Design review of the part shown in the three views and the two pictorial views. Dimensions are in mm from the part's minimum x, y and z. A direction names the side the tool comes from. Give positions to 0.01 mm unless a question says otherwise; leave off trailing zeros. Loops run counter-clockwise (first coordinate to the right, second up) from the corner with the lowest first, then second, coordinate; pieces in that order, holes last. Notation, with made-up numbers: (-21, 14) -> (-14, 14) arc R12 cw to (-14, 32) -> close; hole circle Ø5 at (24.5, -15). An arc over 180 degrees is marked (long way). Use CSV: the item, a comma, the result in double quotes. Start each with the question number.
Item 1: We need section B-B (y = 36). State the section outline as (x, z) points, plus the area to 3 significant figures.
Item 2: Wall thickness on line 1 along X through (y, z) = (45.72, 11.25); line 2 along X through (y, z) = (18.5, 1.75): over which ranges is each line inside the solid? List them lowest first. Write a range as from..to.
Item 3: We need section D-D (x = 45.72). State the section outline as (y, z) points, plus the area to 3 significant figures.
Item 4: We need section C-C (z = 14). Count the separate pieces of the cut face and the enclosed holes in it, plus the area to 3 significant figures.
Item 5: The part is to be moulded in two halves that separate along X. For the marked faces 1, 2, 3 and 4, say which applies: +X half, -X half, draft (parallel to the pull), parting line (faces both ways), or undercut.
Item 6: For the marked faces 5 and 6, list the 3-axis set-ups (+Z, -Z, +X, -X, +Y, -Y) from which the entire face can be reached by the end or side of a thin tool; tool diameter is ignored.
Item 7: We need section A-A (x = 22.4). State the section outline as (y, z) points.
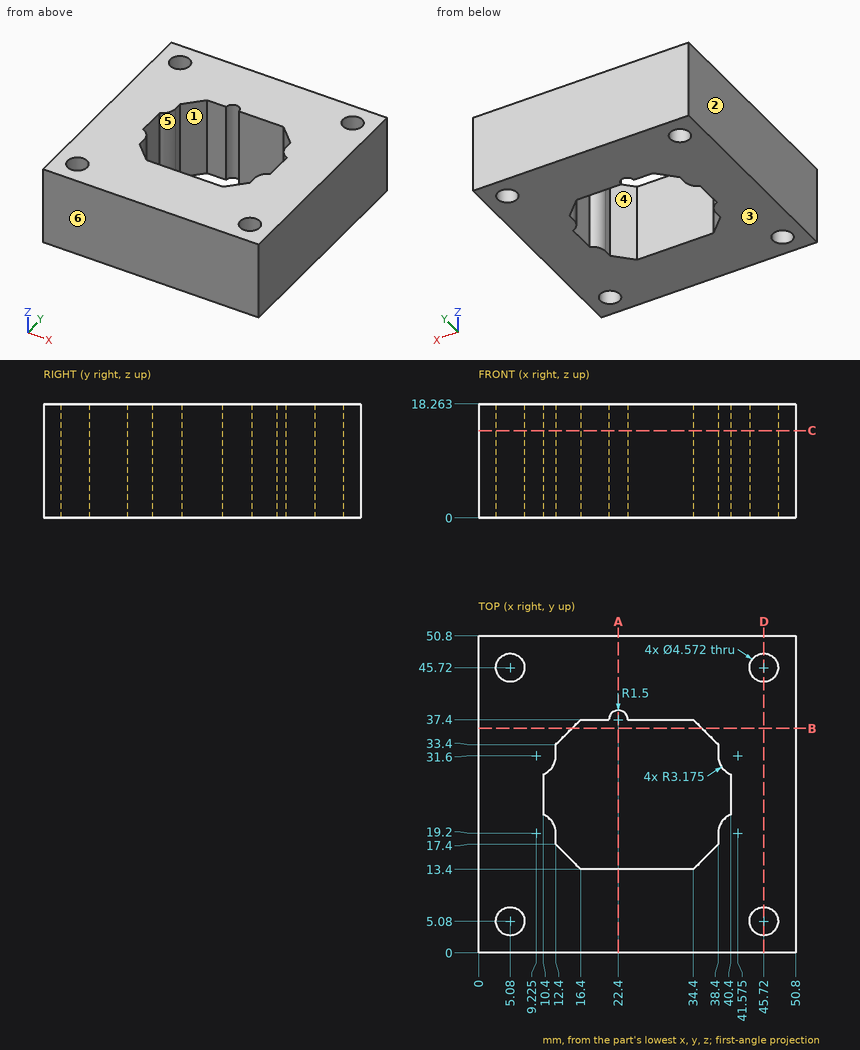
Results found:
1,outline,"(0, 0) -> (15, 0) -> (15, 18.26) -> (0, 18.26) -> close; (35.8, 0) -> (50.8, 0) -> (50.8, 18.26) -> (35.8, 18.26) -> close"
1,area,"548 mm²"
2,line 1,"0..2.79, 7.37..43.43, 48.01..50.8"
2,line 2,"0..12.4, 38.4..50.8"
3,outline,"(0, 0) -> (2.79, 0) -> (2.79, 18.26) -> (0, 18.26) -> close; (7.37, 0) -> (43.43, 0) -> (43.43, 18.26) -> (7.37, 18.26) -> close; (48.01, 0) -> (50.8, 0) -> (50.8, 18.26) -> (48.01, 18.26) -> close"
3,area,"761 mm²"
4,separate pieces,"1"
4,enclosed holes,"5"
4,area,"1,890 mm²"
5,face 1,"undercut"
5,face 2,"-X half"
5,face 3,"draft"
5,face 4,"undercut"
6,face 5,"+Z, -Z"
6,face 6,"+Z, -Z, +X, -X, -Y"
7,outline,"(0, 0) -> (13.4, 0) -> (13.4, 18.26) -> (0, 18.26) -> close; (38.9, 0) -> (50.8, 0) -> (50.8, 18.26) -> (38.9, 18.26) -> close"
